from build123d import *

# Parameters (mm, degrees)
SKETCH1_W           = 164
SKETCH1_H           = 145.68
BOSS_EXTRUDE1_DEPTH = 3
SKETCH2_W           = 164
SKETCH2_H           = 145.68
SKETCH2_W_2         = 154.794377853
SKETCH2_H_2         = 141.122884214
BOSS_EXTRUDE2_DEPTH = 96
SKETCH4_RX          = 60.571165747
SKETCH4_RY          = 25.38547853
CUT_EXTRUDE1_DEPTH  = 20
SKETCH6_W           = 39.790164022
SKETCH6_H           = 75.651590962
CUT_EXTRUDE3_DEPTH  = 20
SKETCH8_W           = 49.5692413
SKETCH8_H           = 91.849069086
BOSS_EXTRUDE3_DEPTH = 32
SKETCH7_W           = 45
SKETCH7_H           = 87.31
CUT_EXTRUDE4_DEPTH  = 32.17
SKETCH9_W           = 11.79717637
SKETCH9_H           = 31.86635219
CUT_EXTRUDE5_DEPTH  = 40
SKETCH11_W          = 16.650134538
SKETCH11_H          = 74.314635754
SKETCH11_W_2        = 24.505886262
CUT_EXTRUDE7_DEPTH  = 40
SKETCH12_R          = 1.77
SKETCH12_R_2        = 1.774021332
CUT_EXTRUDE8_DEPTH  = 40
SKETCH13_R          = 3.893526171
CUT_EXTRUDE9_DEPTH  = 40


with BuildPart() as part:
    # Sketch1 → Boss-Extrude1 (new body)
    with BuildSketch(Plane(origin=(0, 0, 0), x_dir=(1, 0, 0), z_dir=(0, 1, 0))):
        with Locations((9.099573667, 28.508659662)):
            Rectangle(SKETCH1_W, SKETCH1_H)
    extrude(amount=BOSS_EXTRUDE1_DEPTH)

    # Sketch2 → Boss-Extrude2 (add)
    with BuildSketch(Plane(origin=(0, 3, 0), x_dir=(1, 0, 0), z_dir=(0, 1, 0))):
        with Locations((9.099573667, 28.508659662)):
            Rectangle(SKETCH2_W, SKETCH2_H)
        with Locations((6.2438887, 28.265919971)):
            Rectangle(SKETCH2_W_2, SKETCH2_H_2, mode=Mode.SUBTRACT)
    extrude(amount=BOSS_EXTRUDE2_DEPTH)

    # Sketch4 → Cut-Extrude1 (cut)
    with BuildSketch(Plane(origin=(91.099573667, 0, 0), x_dir=(0, 0, -1), z_dir=(1, 0, 0))):
        with Locations(Location((28.714709394, 51.858345631), (0, 0, -3.107007487))):
            Ellipse(SKETCH4_RX, SKETCH4_RY)
    extrude(amount=-CUT_EXTRUDE1_DEPTH, mode=Mode.SUBTRACT)

    # Sketch6 → Cut-Extrude3 (cut)
    with BuildSketch(Plane.ZY.offset(72.900426333)):
        with Locations((19.353212204, 44.793227562)):
            Rectangle(SKETCH6_W, SKETCH6_H)
    extrude(amount=-CUT_EXTRUDE3_DEPTH, mode=Mode.SUBTRACT)

    # Sketch8 → Boss-Extrude3 (add)
    with BuildSketch(Plane(origin=(0, 3, 0), x_dir=(1, 0, 0), z_dir=(0, 1, 0))):
        with Locations((5.315093732, 20.62475692)):
            Rectangle(SKETCH8_W, SKETCH8_H)
    extrude(amount=BOSS_EXTRUDE3_DEPTH)

    # Sketch7 → Cut-Extrude4 (cut)
    with BuildSketch(Plane.XZ):
        with Locations((5.233997278, -20.691377503)):
            Rectangle(SKETCH7_W, SKETCH7_H)
    extrude(amount=-CUT_EXTRUDE4_DEPTH, mode=Mode.SUBTRACT)

    # Sketch9 → Cut-Extrude5 (cut)
    with BuildSketch(Plane.XZ.offset(-32.17)):
        with Locations((-9.959298471, -44.905011983)):
            Rectangle(SKETCH9_W, SKETCH9_H)
    extrude(amount=-CUT_EXTRUDE5_DEPTH, mode=Mode.SUBTRACT)

    # Sketch11 → Cut-Extrude7 (cut)
    with BuildSketch(Plane.XZ):
        with Locations((50.891184892, -21.453909531)):
            Rectangle(SKETCH11_W, SKETCH11_H)
        with Locations((-43.781754887, -21.453909531)):
            Rectangle(SKETCH11_W_2, SKETCH11_H)
    extrude(amount=-CUT_EXTRUDE7_DEPTH, mode=Mode.SUBTRACT)

    # Sketch12 → Cut-Extrude8 (cut)
    with BuildSketch(Plane(origin=(91.099573667, 0, 0), x_dir=(0, 0, -1), z_dir=(1, 0, 0))):
        with Locations((37.87743885, 91.391738709)):
            Circle(SKETCH12_R)
        with Locations((14.300129623, 91.391738709)):
            Circle(SKETCH12_R_2)
    extrude(amount=-CUT_EXTRUDE8_DEPTH, mode=Mode.SUBTRACT)

    # Sketch13 → Cut-Extrude9 (cut)
    with BuildSketch(Plane.XZ):
        with Locations((-59.534784008, -89.003983448)):
            Circle(SKETCH13_R)
    extrude(amount=-CUT_EXTRUDE9_DEPTH, mode=Mode.SUBTRACT)


solid = part.part
Build history of the part. All positions in model axes, mm. A direction names the side the tool comes from. Give positions to 0.01 mm unless a question says otherwise; leave off trailing zeros. Order: outer loops, then holes, each group sorted by start corner. A loop starts at its lowest first (then second) coordinate and runs counter-clockwise, first axis right, second up. Notation, with made-up numbers: M 11,43.5 L 28,43.5 A23 ccw 28,71.5 Z; hole C 67.25,-38 d2. An arc over 180 degrees is marked long. Put each result on its own line as item: value.
Item 1: Slice it at B-B, the plane x = 52.5. Write the cut outline in (y, z).
From the geometry:
outline: M 0,-101.35 L 99,-101.35 L 99,-98.83 L 3,-98.83 L 3,-58.61 L 0,-58.61 Z; M 0,15.7 L 3,15.7 L 3,42.3 L 99,42.3 L 99,44.33 L 0,44.33 Z
Item 2: Two-plate mould, pull along Z, no slides. Class faces 1 (the flat face through (5, 50, -98.827)), 2 (the flat face through (45, 99, -99)), 3 (the flat face through (8, 49, 44.331)): +Z half, -Z half, draft (parallel to the pull), parting line (faces both ways), or undercut.
From the geometry:
face 1: undercut
face 2: draft
face 3: +Z half
Item 3: Slice it at C-C, the plane y = 86. Write the cut outline in (x, z).
From the geometry:
outline: M -72.9,-101.35 L 91.1,-101.35 L 91.1,44.33 L -72.9,44.33 Z; hole M -71.15,-98.83 L 83.64,-98.83 L 83.64,42.3 L -71.15,42.3 Z
Item 4: 3-axis set-ups, long thin cutter, end or side, ignore diameter. For faces 4 (the flat face through (91.1, 27, -11)), 5 (the flat face through (-71.153, 50, -43)), 6 (the flat face through (5, 16, 22.964)): which of +Z, -Z, +X, -X, +Y, -Y reach the whole face in a straight line?
From the geometry:
face 4: +Z, -Z, +X, +Y, -Y
face 5: +Y
face 6: -Y
Item 5: Slice it at D-D, the plane x = 7.5. Write the cut outline in (y, z).
From the geometry:
outline: M 0,-101.35 L 99,-101.35 L 99,-98.83 L 3,-98.83 L 3,-66.55 L 35,-66.55 L 35,25.3 L 3,25.3 L 3,42.3 L 99,42.3 L 99,44.33 L 0,44.33 L 0,22.96 L 32.17,22.96 L 32.17,-64.35 L 0,-64.35 Z
Item 6: Slice it at A-A, the plane y = 14. Write the cut outline in (x, z), plus the area to 3 significant figures.
From the geometry:
outline: M -72.9,-101.35 L 91.1,-101.35 L 91.1,44.33 L -72.9,44.33 L -72.9,39.25 L -71.15,39.25 L -71.15,42.3 L 83.64,42.3 L 83.64,-98.83 L -71.15,-98.83 L -71.15,-0.54 L -72.9,-0.54 Z; M -19.47,-66.55 L 30.1,-66.55 L 30.1,25.3 L -19.47,25.3 Z; hole M -17.27,-64.35 L 27.73,-64.35 L 27.73,22.96 L -17.27,22.96 Z
area: 2,600 mm2
Item 7: Flat gauge pin, fed straight in: pin 1 Ø5 at (y, z) = (25.5, 8) entering from -X. Where does the tip first touch, or does it go through?
From the geometry:
pin 1: stops at x = -19.47
Item 8: Probe line 1 (X direction, y = 28.5, z = 21.5); line 2 (Z direction, x = -33, y = 70); line 3 (X direction, y = 18.5, z = -27). List the from-to ranges inside material, lowest first. Write a range as [from, to].
From the geometry:
line 1: x = [-19.47, -17.27], [27.73, 30.1], [83.64, 91.1]
line 2: z = [-101.35, -98.83], [42.3, 44.33]
line 3: x = [-72.9, -71.15], [-19.47, -17.27], [27.73, 30.1], [83.64, 91.1]
